The listing builds one solid part. Answer for the finished solid, in the listing's coordinates (mm). Face numbers are marked on the shaded views. Give positions to 0.01 mm unless a question says otherwise; leave off trailing zeros. Loops run counter-clockwise (first coordinate to the right, second up) from the corner with the lowest first, then second, coordinate; pieces in that order, holes last. Notation, with made-up numbers: (45, -29) - (82, -29) arc R14 cw to (82, -21) - close; hole circle Ø4 at (-7, 69). An arc over 180 degrees is marked (long way). Write each question's results on one line, items separated by ' | '.
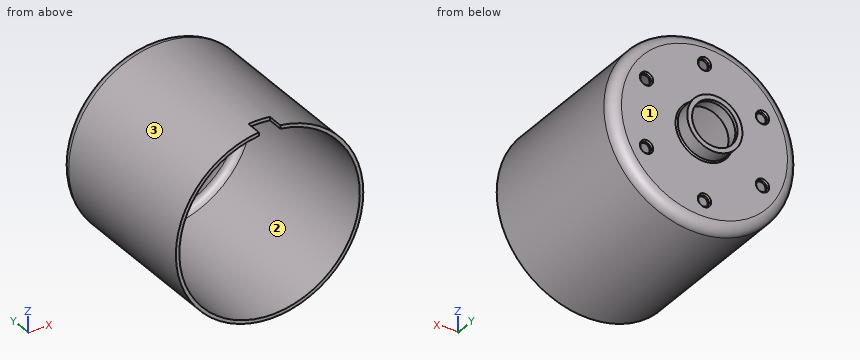
from build123d import *

# Parameters (mm, degrees)
SKETCH1_R                    = 17.5
BOSS_EXTRUDE1_DEPTH          = 33
FILLET1_R                    = 2
SKETCH3_R                    = 5.15
BOSS_EXTRUDE2_DEPTH          = 3
CHAMFER1_SIZE                = 0.25
SHELL1_T                     = -0.65
CUT_EXTRUDE1_REACH           = 45.686
SKETCH4_R                    = 4.25
CUT_EXTRUDE2_REACH           = 43.249
SKETCH5_R                    = 1
CHAMFER2_SIZE                = 0.25
CIRPATTERN1_COUNT            = 6
CHAMFER2_OF_CIRPATTERN1_SIZE = 0.25
CUT_EXTRUDE3_REACH           = 55.172
CUT_EXTRUDE3_END_RADIUS      = 16.85
SKETCH6_W                    = 4
SKETCH6_H                    = 6


with BuildPart() as part:
    # Sketch1 → Boss-Extrude1 (new body)
    with BuildSketch(Plane(origin=(0, 0, 0), x_dir=(1, 0, 0), z_dir=(0, 1, 0))):
        with Locations(Location((0, 0, 0), (0, 0, 270))):
            Circle(SKETCH1_R)
    extrude(amount=BOSS_EXTRUDE1_DEPTH)

    # Fillet1
    fillet1_edges = [part.edges().sort_by_distance(p)[0] for p in [
        (0, 33, -17.5),
    ]]
    fillet(fillet1_edges, radius=FILLET1_R)

    # Sketch3 → Boss-Extrude2 (add)
    with BuildSketch(Plane(origin=(0, 33, 0), x_dir=(1, 0, 0), z_dir=(0, 1, 0))):
        with Locations(Location((0, 0, 0), (0, 0, 270))):
            Circle(SKETCH3_R)
    extrude(amount=BOSS_EXTRUDE2_DEPTH)

    # Chamfer1
    chamfer1_edges = [part.edges().sort_by_distance(p)[0] for p in [
        (0, 33, -5.15),
    ]]
    chamfer(chamfer1_edges, length=CHAMFER1_SIZE)

    # Shell1
    shell1_openings = [part.faces().sort_by_distance(p)[0] for p in [
        (0, 0, 0),
    ]]
    offset(amount=SHELL1_T, openings=shell1_openings, kind=Kind.INTERSECTION)

    # Sketch4 → Cut-Extrude1 (cut, up to next)
    with BuildSketch(Plane(origin=(0, 36, 0), x_dir=(1, 0, 0), z_dir=(0, 1, 0)), mode=Mode.PRIVATE) as cut_extrude1_sk1:
        with Locations(Location((0, 0, 0), (0, 0, 270))):
            Circle(SKETCH4_R)
    cut_extrude1_tool1 = extrude(cut_extrude1_sk1.sketch, amount=-CUT_EXTRUDE1_REACH, mode=Mode.PRIVATE) & part.part
    add(cut_extrude1_tool1.solids().sort_by_distance((0, 36, 0))[0], mode=Mode.SUBTRACT)

    # Sketch5 → Cut-Extrude2 (cut, up to next)
    with BuildSketch(Plane(origin=(0, 33, 0), x_dir=(1, 0, 0), z_dir=(0, 1, 0)), mode=Mode.PRIVATE) as cut_extrude2_sk1:
        with Locations(Location((0, 12.5, 0), (0, 0, 270))):
            Circle(SKETCH5_R)
    cut_extrude2_tool1 = extrude(cut_extrude2_sk1.sketch, amount=-CUT_EXTRUDE2_REACH, mode=Mode.PRIVATE) & part.part
    cut_extrude2 = cut_extrude2_tool1.solids().sort_by_distance((0, 33, -12.5))[0]
    add(cut_extrude2, mode=Mode.SUBTRACT)

    # Chamfer2
    chamfer2_edges = [part.edges().sort_by_distance(p)[0] for p in [
        (0, 33, -13.5),
    ]]
    chamfer(chamfer2_edges, length=CHAMFER2_SIZE)

    # CirPattern1: Cut-Extrude2 ×6 about axis
    cirpattern1_axis = Axis((0, 0, 0), (0, 1, 0))
    for i in range(1, CIRPATTERN1_COUNT):
        add(cut_extrude2.rotate(cirpattern1_axis, i * 360 / CIRPATTERN1_COUNT), mode=Mode.SUBTRACT)

    # Chamfer2 of CirPattern1
    chamfer2_of_cirpattern1_edges = [part.edges().sort_by_distance(p)[0] for p in [
        (-11.691342951, 33, -6.75),
        (-11.691342951, 33, 6.75),
        (0, 33, 13.5),
        (11.691342951, 33, 6.75),
        (11.691342951, 33, -6.75),
    ]]
    chamfer(chamfer2_of_cirpattern1_edges, length=CHAMFER2_OF_CIRPATTERN1_SIZE)

    # Cut-Extrude3: up to this cylinder (the profile starts outside it)
    cut_extrude3_end = Plane(origin=(0, 0, 0), z_dir=(0, -1, 0)) * Cylinder(CUT_EXTRUDE3_END_RADIUS, 145.044, mode=Mode.PRIVATE)
    # Sketch6 → Cut-Extrude3 (cut, up to the surface)
    with BuildSketch(Plane.XY.offset(17.5), mode=Mode.PRIVATE) as cut_extrude3_sk1:
        Rectangle(SKETCH6_W, SKETCH6_H)
    cut_extrude3_tool1 = extrude(cut_extrude3_sk1.sketch, amount=-CUT_EXTRUDE3_REACH, mode=Mode.PRIVATE) - cut_extrude3_end
    add(cut_extrude3_tool1.solids().sort_by_distance((0, 0, 17.5))[0], mode=Mode.SUBTRACT)


solid = part.part
Item 1: Flat-ended cylindrical pins translate along their axes: P1, Ø10, axis at x = 12, y = 18.5, coming from the +Z side; P2, Ø6, axis at y = 5, z = -8.5, coming from the +X side; P3, Ø1.5, axis at x = -6, y = 23.5, coming from the +Z side; P4, Ø8, axis at x = 0, z = 0, coming from the +Y side. Find the tip coordinate at first contact, or state that the pin passes through.
Values found:
P1: stops at z = 16.04 | P2: stops at x = 16.61 | P3: stops at z = 16.69 | P4: passes through
Item 2: A cutting plane is placed at B-B, the plane y = 21. Determine the outline of the cut face in (x, z), plus the area to 3 significant figures.
Values found:
outline: circle Ø35 at (0, 0); hole circle Ø33.7 at (0, 0) | area: 70.1 mm²
Item 3: A cutting plane is placed at A-A, the plane z = 0. Determine the outline of the cut face in (x, y).
Values found:
outline: (-17.5, 0) - (-16.85, 0) - (-16.85, 31) arc R1.35 cw to (-15.5, 32.35) - (-5.13, 32.35) - (-4.5, 32.98) - (-4.5, 35.35) - (-4.25, 35.35) - (-4.25, 36) - (-5.15, 36) - (-5.15, 33.25) - (-5.4, 33) - (-15.5, 33) arc R2 ccw to (-17.5, 31) - close; (4.25, 35.35) - (4.5, 35.35) - (4.5, 32.98) - (5.13, 32.35) - (15.5, 32.35) arc R1.35 cw to (16.85, 31) - (16.85, 0) - (17.5, 0) - (17.5, 31) arc R2 ccw to (15.5, 33) - (5.4, 33) - (5.15, 33.25) - (5.15, 36) - (4.25, 36) - close
Item 4: A cutting plane is placed at C-C, the plane x = 0. Count the separate pieces of the cut face and the enclosed holes in it, plus the area to 3 significant figures.
Values found:
separate pieces: 4 | enclosed holes: 0 | area: 57.2 mm²
Item 5: For a pull along Z with two mould halves and no side action, classify the marked faces 1, 2 and 3 as released by +Z, released by -Z, zero draft, split by the parting line, or undercut.
Values found:
face 1: zero draft | face 2: undercut | face 3: split by the parting line
Item 6: Find the intervals of material crossed by line 1 along X through (y, z) = (32.5, 12.5); line 2 along X through (y, z) = (32.6, 6.25); line 3 along Y through (x, z) = (1.5, -14), in increasing order. Write a range as [from, to].
Values found:
line 1: x = [-11.26, -1], [1, 11.26] | line 2: x = [-15.49, -11.83], [-9.83, 9.83], [11.83, 15.49] | line 3: y = [32.35, 33]
